Check sheet for the modelled part. Datum: model origin and axes. Units: mm. Face numbers are marked on the shaded views. A direction names the side the tool comes from. Give positions to 0.01 mm unless a question says otherwise; leave off trailing zeros. Order: outer loops, then holes, each group sorted by start corner. A loop starts at its lowest first (then second) coordinate and runs counter-clockwise, first axis right, second up. Notation, with made-up numbers: (76, 71.25) -> (85, 71.25) arc R31 cw to (85, 97.25) -> close; hole circle Ø9 at (-8.75, -9). An arc over 180 degrees is marked (long way). Write each question's results on one line, items separated by ' | '.
Autodesk Inventor part; units mm, degrees
ref_plane "YZ Plane" through (0, 0, 0) normal (1, 0, 0) x (0, 1, 0)
ref_plane "XZ Plane" through (0, 0, 0) normal (0, 1, 0) x (-1, 0, 0)
ref_plane "XY Plane" through (0, 0, 0) normal (0, 0, 1) x (1, 0, 0)
sketch "Sketch1" plane through (0, 0, 0) normal (0, 0, 1) x (1, 0, 0)
  line L0 (0, 0) -> (80, 0)
  line L1 (80, 0) -> (80, 100)
  line L2 (80, 100) -> (0, 100)
  line L3 (0, 100) -> (0, 0)
  dimension "d0" = 80
  dimension "d1" = 100
extrude "Plate1" add sketch "Sketch1" along normal blind 0.5
sketch "Sketch2" plane through (0, 99.6464, 0.3536) normal (0, 0.7071068, -0.7071068) x (-1, 0, 0)
  line L0 (-80, 0) -> (0, 0)
  line L1 (0, 0) -> (0, 200)
  line L2 (0, 200) -> (-80, 200)
  line L3 (-80, 200) -> (-80, 0)
edge flange "Flange1" height 200 angle 45 thickness 0.5 bend radius 0.5 thickness toward (0, 0.7071068, -0.7071068) relief tear relief width 0.5 relief depth 0.25 edges at (40, 100, 0.5) wall of the first edge with corners at (80, 99.6464, 0.3536) (0, 99.6464, 0.3536) (0, 241.0678, 141.7749) (80, 241.0678, 141.7749)
bend "Bend1"
corner "Corner1"
equation "\"d3\" = BendReliefWidth"
equation "\"d4\" = BendReliefDepth"
equation "\"d5\" = MinimumRemnant"
equation "\"d6\" = BendRadius"
equation "\"d9\" = BendRadius"
equation "\"d10\" = CornerReliefSize"
equation "\"d11\" = GapSize"
equation "\"d12\" = JacobiRadiusSize"
equation "\"BendRadius\" = Thickness"
equation "\"BendReliefWidth\" = Thickness"
equation "\"BendReliefDepth\" = 0.5 * Thickness"
equation "\"CornerReliefSize\" = 4 * Thickness"
equation "\"MinimumRemnant\" = 2 * Thickness"
equation "\"TransitionRadius\" = BendRadius"
equation "\"JacobiRadiusSize\" = BendRadius"
equation "\"GapSize\" = Thickness"
equation "\"d2\" = BendRadius"
properties part number "Tunel_GridPlate" material "Stainless Steel"
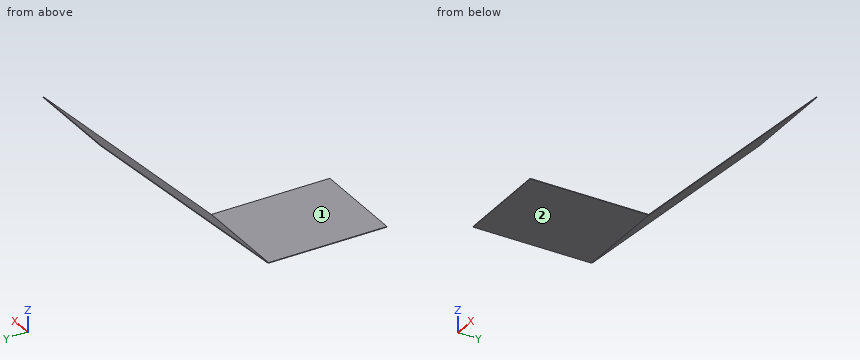
1. Material ranges on probe 1 along Z at (x, y) = (47, 51.5); probe 2 along Z at (x, y) = (34.5, 138.5); probe 3 along Y at (x, z) = (10, 109.5), recorded low to high. Write a range as from..to.
Verdict:
probe 1: z = 0..0.5 | probe 2: z = 38.5..39.21 | probe 3: y = 208.79..209.5
2. Section check A-A on x = 39. Record the cut outline in (y, z).
Verdict:
outline: (0, 0) -> (99.59, 0) arc R1 ccw to (100.29, 0.29) -> (241.42, 141.42) -> (241.07, 141.77) -> (99.94, 0.65) arc R0.5 cw to (99.59, 0.5) -> (0, 0.5) -> close
3. Section check C-C on z = 52. Record the cut outline in (x, y).
Verdict:
outline: (0, 151.29) -> (80, 151.29) -> (80, 152) -> (0, 152) -> close
4. Section check B-B on y = 66.5. Record the cut outline in (x, z), then the cut area to 3 significant figures.
Verdict:
outline: (0, 0) -> (80, 0) -> (80, 0.5) -> (0, 0.5) -> close | area: 40.0 mm^2
5. Access from +Z, -Z, +X, -X, +Y, -Y to the whole of each face (thin tool, end or side, straight path). Record for the marked faces 1 and 2.
Verdict:
face 1: +Z, +X, -X, -Y | face 2: -Z, +X, -X, +Y, -Y
6. Gauge pin test, flat ends, axial feed: pin 1 Ø12 at (x, z) = (12, 106.5) entering from +Y; pin 2 Ø5 at (x, z) = (52, 35.5) entering from -Y; pin 3 Ø3 at (x, z) = (58, 55.5) entering from -Y; pin 4 Ø6 at (y, z) = (133, 26) entering from -X. Record the tip position at first contact, or that the pin passes through.
Verdict:
pin 1: stops at y = 212.5 | pin 2: stops at y = 132.29 | pin 3: stops at y = 153.29 | pin 4: passes through
